```python
from build123d import *

# Parameters (mm, degrees)
F0_W     = 91.2344232202
F0_H     = 83.7330448863
F1_DEPTH = 8.128
F0_H_2   = 14.015381963
F2_DEPTH = 17.018
F3_T     = -1.9304
F4_D     = 6.2484


# Not quite as in the source:
# - a shell that OpenCascade refuses in one call is made with other operations: the cavity is built on its own and cut out


with BuildPart() as f1:
    # F0 (on Top) → F1 (new body)
    with BuildSketch(Plane.XY):
        with Locations((-8.2024671137, 9.545179052)):
            Rectangle(F0_W, F0_H)
    extrude(amount=F1_DEPTH)

    # F0 (on Top) → F2 (join)
    with BuildSketch(Plane.XY):
        with Locations((-8.2024671137, -39.3290343727)):
            Rectangle(F0_W, F0_H_2)
    extrude(amount=F2_DEPTH)

    # F3: a shell. OpenCascade refuses it in one call, so the cavity is built on its own and cut out:
    # the body offset inwards by the wall thickness, plus a prism from it out through each open face.
    f3_core = offset(f1.part, amount=F3_T, kind=Kind.INTERSECTION, mode=Mode.PRIVATE)
    f3_exits = [f3_core.faces().sort_by_distance(p)[0] for p in [
        (-8.202467, -34.251743, 10.6426),
    ]]
    add(f3_core, mode=Mode.SUBTRACT)
    extrude(f3_exits, amount=-F3_T, mode=Mode.SUBTRACT)

    # F4 (through all)
    with Locations(Plane(origin=(0, 0, 0), x_dir=(1, 0, 0), z_dir=(0, 0, -1))):
        with Locations((37.4147444963, 46.3367253542), (-53.8196787238, 46.3367253542)):
            Hole(F4_D / 2)


solid = f1.part
```
Work out the finished part from the listing and answer in its coordinate system (mm). A direction names the side the tool comes from. Give positions to 0.01 mm unless a question says otherwise; leave off trailing zeros. Write each loop counter-clockwise with the first axis right and the second up, starting at its lowest first coordinate (ties: lowest second). Pieces come first, ordered by that corner, then holes. Notation, with made-up numbers: (36.5, 23.25) -> (88.5, 23.25) arc R34 cw to (88.5, 56.25) -> close; hole circle Ø4 at (-16.75, -26). An arc over 180 degrees is marked (long way). Write item = value, one per line.
Q1. A tool of negligible diameter and unlimited length cuts with its end or side. For faces 4 (the flat face through (-51.889, -8, 6)), 5 (the flat face through (-9, -38, 15.088)), 6 (the flat face through (-9, 49.481, 4)), 7 (the flat face through (-8, -32.321, 16)), 8 (the flat face through (-9, -44.406, 8)), from which of +Z, -Z, +X, -X, +Y, -Y can it reach the whole face along a straight path? Write none if from no direction.
Computed values:
face_4 = -Y
face_5 = +Y
face_6 = none
face_7 = +Z, +X, -X, +Y
face_8 = +X, -X
Q2. Section B-B on y = -27 is taken. Determine the outline of the cut face in (x, z).
Computed values:
outline = (-53.82, 0) -> (37.41, 0) -> (37.41, 8.13) -> (-53.82, 8.13) -> close; hole (-51.89, 1.93) -> (35.48, 1.93) -> (35.48, 6.2) -> (-51.89, 6.2) -> close
Q3. Section D-D on x = 14 is taken. Determine the outline of the cut face in (y, z), and give its area (3 significant figures).
Computed values:
outline = (-46.34, 0) -> (51.41, 0) -> (51.41, 8.13) -> (-32.32, 8.13) -> (-32.32, 6.2) -> (49.48, 6.2) -> (49.48, 1.93) -> (-44.41, 1.93) -> (-44.41, 15.09) -> (-32.32, 15.09) -> (-32.32, 17.02) -> (-46.34, 17.02) -> close
area = 411 mm^2
Q4. Section C-C on z = 10 is taken. Determine the outline of the cut face in (x, y).
Computed values:
outline = (-53.82, -43.21) arc R3.12 cw to (-51.89, -43.88) -> (-51.89, -32.32) -> (-53.82, -32.32) -> close; (-51.36, -44.41) arc R3.12 cw to (-50.7, -46.34) -> (34.29, -46.34) arc R3.12 cw to (34.96, -44.41) -> close; (35.48, -43.88) arc R3.12 cw to (37.41, -43.21) -> (37.41, -32.32) -> (35.48, -32.32) -> close
Q5. Consider line 1 along Z through (x, y) = (-19, 27); line 2 along X through (y, z) = (7.5, 5.75); line 3 along Y through (x, z) = (11, 3.5). Determine where each line is inside the solid, lowest interval first.
Computed values:
line_1 = 0 to 1.93, 6.2 to 8.13
line_2 = -53.82 to -51.89, 35.48 to 37.41
line_3 = -46.34 to -44.41, 49.48 to 51.41
Q6. Section A-A on z = 3.5 is taken. Determine the outline of the cut face in (x, y).
Computed values:
outline = (-53.82, -43.21) arc R3.12 cw to (-51.89, -43.88) -> (-51.89, 49.48) -> (35.48, 49.48) -> (35.48, -43.88) arc R3.12 cw to (37.41, -43.21) -> (37.41, 51.41) -> (-53.82, 51.41) -> close; (-51.36, -44.41) arc R3.12 cw to (-50.7, -46.34) -> (34.29, -46.34) arc R3.12 cw to (34.96, -44.41) -> close
Q7. Flat-ended cylindrical pins translate along their axes: pin 1 Ø2 at (x, y) = (-15.5, -25.5) entering from +Z; pin 2 Ø10 at (x, z) = (12, 11.5) entering from +Y. Find the tip coordinate at first contact, or state that the pin passes through.
Computed values:
pin_1 = 8.13
pin_2 = 51.41
Q8. For a pull along Y with two mould halves and no side action, classify faces 1 (the flat face through (-9, 3, 1.93)), 2 (the flat face through (-9, 10, 8.128)), 3 (the flat face through (-9, 51.412, 4)) as pulls with the +Y half, pulls with the -Y half, needs draft (parallel to the pull), parting line crosses it, or undercut.
Computed values:
face_1 = undercut
face_2 = needs draft
face_3 = pulls with the +Y half
